The listing builds one solid part. Answer for the finished solid, in the listing's coordinates (mm). Face numbers are marked on the shaded views. A direction names the side the tool comes from. Round coordinates to 2 decimals unless told otherwise and drop trailing zeros.
(1) The mould has two halves that part along Y. Classify the marked faces 1, 2 and 3: +Y half, -Y half, draft (parallel to the pull), parting line (faces both ways), or undercut.
(2) Each of these flat-tipped pins is pushed along its axis until it touches: pin 1 Ø3 at (x, z) = (52, 11) entering from +Y; pin 2 Ø6 at (y, z) = (187, 3) entering from +X; pin 3 Ø6 at (y, z) = (240.5, 4) entering from -X. Where does it stop, or does it pass through?
(3) Find the intervals of material crossed by probe 1 along Y at (x, z) = (65, 4.5); probe 2 along X at (y, z) = (166, 11); probe 3 along X at (y, z) = (217.5, 1.5), in increasing order.
(4) A cutting plane is placed at A-A, the plane y = 163. Give the number of separate pieces and of enclosed holes in the cut face, and give its area (3 significant figures).
(5) For the marked faces 4 and 5, determine the directions among +Z, -Z, +X, -X, +Y, -Y from which every point of the face is accessible in a straight line to the end or side of a thin tool.
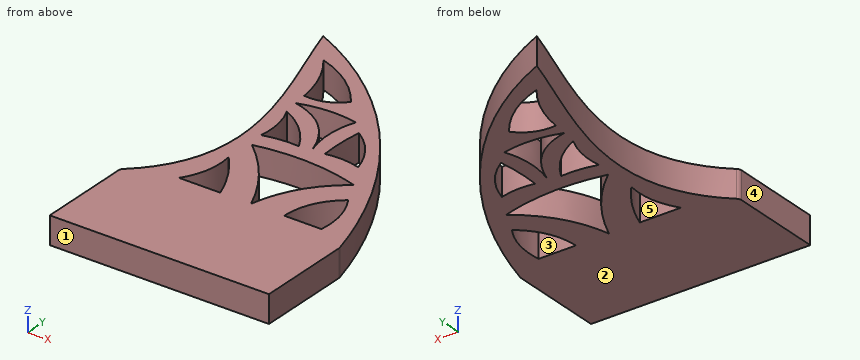
from build123d import *

# Parameters (mm, degrees)
SKETCH1_W           = 101.6
SKETCH1_H           = 152.4
BOSS_EXTRUDE1_DEPTH = 12.7
BOSS_EXTRUDE3_DEPTH = 12.7
FILLET1_R           = 2.54
FILLET2_R           = 5.08
CUT_EXTRUDE1_DEPTH  = 298.570512784


with BuildPart() as part:
    # Sketch1 → Boss-Extrude1 (new body)
    with BuildSketch(Plane.XY):
        with Locations((50.8, 76.2)):
            Rectangle(SKETCH1_W, SKETCH1_H)
    extrude(amount=BOSS_EXTRUDE1_DEPTH)

    # Sketch2 → Boss-Extrude3 (add)
    with BuildSketch(Plane.XY):
        with BuildLine():
            add(Edge.make_bspline(
                [(0, 152.4), (39.790111277, 186.839065643), (12.30975625, 238.845497073), (0, 279.4)],
                knots=[0, 0, 0, 0, 1, 1, 1, 1], degree=3))
            add(Edge.make_bspline(
                [(0, 279.4), (51.286050257, 256.550041835), (87.836892382, 205.957944637), (101.6, 152.4)],
                knots=[0, 0, 0, 0, 1, 1, 1, 1], degree=3))
            Line((101.6, 152.4), (0, 152.4))
        make_face()
        with BuildLine():
            add(Edge.make_bspline(
                [(49.225838487, 233.315766274), (35.641228944, 236.267866949), (22.375615267, 231.937259722)],
                knots=[0, 0, 0, 1, 1, 1], degree=2))
            add(Edge.make_bspline(
                [(48.400350721, 207.535437601), (42.054170901, 227.566198031), (22.375615267, 231.937259722)],
                knots=[0, 0, 0, 1, 1, 1], degree=2))
            add(Edge.make_bspline(
                [(48.400350721, 207.535437601), (44.393568943, 220.734513873), (49.225838487, 233.315766274)],
                knots=[0, 0, 0, 1, 1, 1], degree=2))
        make_face(mode=Mode.SUBTRACT)
        with BuildLine():
            add(Edge.make_bspline(
                [(43.05348098, 206.08803494), (36.239789994, 218.91266054), (23.516066372, 224.861937296)],
                knots=[0, 0, 0, 1, 1, 1], degree=2))
            add(Edge.make_bspline(
                [(23.516066372, 224.861937296), (28.235295407, 215.21927262), (26.605728117, 204.582177714)],
                knots=[0, 0, 0, 1, 1, 1], degree=2))
            add(Edge.make_bspline(
                [(26.605728117, 204.582177714), (34.700432609, 206.792891754), (43.05348098, 206.08803494)],
                knots=[0, 0, 0, 1, 1, 1], degree=2))
        make_face(mode=Mode.SUBTRACT)
        with BuildLine():
            add(Edge.make_bspline(
                [(82.396089655, 183.81371778), (70.6713649, 174.663598784), (70.32777317, 160.02)],
                knots=[0, 0, 0, 1, 1, 1], degree=2))
            Line((70.32777317, 160.02), (87.546521436, 160.02))
            add(Edge.make_bspline(
                [(82.396089655, 183.81371778), (89.339550367, 172.773814043), (87.546521436, 160.02)],
                knots=[0, 0, 0, 1, 1, 1], degree=2))
        make_face(mode=Mode.SUBTRACT)
        with BuildLine():
            add(Edge.make_bspline(
                [(26.980466376, 183.81374211), (28.958775605, 170.837543608), (21.602944743, 160.02)],
                knots=[0, 0, 0, 1, 1, 1], degree=2))
            Line((21.602944743, 160.02), (40.676641776, 160.02))
            add(Edge.make_bspline(
                [(26.980466376, 183.81374211), (36.13847285, 173.175056715), (40.676641776, 160.02)],
                knots=[0, 0, 0, 1, 1, 1], degree=2))
        make_face(mode=Mode.SUBTRACT)
        with BuildLine():
            add(Edge.make_bspline(
                [(54.97708308, 160.02), (46.08347584, 181.54755316), (28.342136903, 196.529802482)],
                knots=[0, 0, 0, 1, 1, 1], degree=2))
            add(Edge.make_bspline(
                [(28.342136903, 196.529802482), (53.017815002, 201.732288521), (77.187204495, 194.363538628)],
                knots=[0, 0, 0, 1, 1, 1], degree=2))
            add(Edge.make_bspline(
                [(54.97708308, 160.02), (59.374728895, 181.400643158), (77.187204495, 194.363538628)],
                knots=[0, 0, 0, 1, 1, 1], degree=2))
        make_face(mode=Mode.SUBTRACT)
        with BuildLine():
            add(Edge.make_bspline(
                [(70.328259561, 206.277457578), (62.361576962, 208.669014941), (54.287141362, 207.109917469)],
                knots=[0, 0, 0, 1, 1, 1], degree=2))
            add(Edge.make_bspline(
                [(54.287141362, 207.109917469), (53.482096811, 217.391663167), (54.97708308, 227.557269012)],
                knots=[0, 0, 0, 1, 1, 1], degree=2))
            add(Edge.make_bspline(
                [(54.97708308, 227.557269012), (66.645859754, 219.852180834), (70.328259561, 206.277457578)],
                knots=[0, 0, 0, 1, 1, 1], degree=2))
        make_face(mode=Mode.SUBTRACT)
        with BuildLine():
            add(Edge.make_bspline(
                [(21.602944743, 238.323137826), (19.95197567, 252.974545225), (11.094737768, 264.601494061)],
                knots=[0, 0, 0, 1, 1, 1], degree=2))
            add(Edge.make_bspline(
                [(11.094737768, 264.601494061), (28.053835186, 259.295838115), (38.412267282, 244.949944056)],
                knots=[0, 0, 0, 1, 1, 1], degree=2))
            add(Edge.make_bspline(
                [(21.602944743, 238.323137826), (31.864782779, 237.284469605), (38.412267282, 244.949944056)],
                knots=[0, 0, 0, 1, 1, 1], degree=2))
        make_face(mode=Mode.SUBTRACT)
    extrude(amount=BOSS_EXTRUDE3_DEPTH)

    # Fillet1
    fillet1_edges = [part.edges().sort_by_distance(p)[0] for p in [
        (101.6, 152.4, 6.35),
        (0, 152.4, 6.35),
    ]]
    fillet(fillet1_edges, radius=FILLET1_R)

    # Fillet2
    fillet2_edges = [part.edges().sort_by_distance(p)[0] for p in [
        (0, 0, 6.35),
        (101.6, 0, 6.35),
    ]]
    fillet(fillet2_edges, radius=FILLET2_R)

    # Sketch4 → Cut-Extrude1 (cut, through all)
    with BuildSketch(Plane.XY.offset(12.7)):
        Polygon((101.519048921, 108.263964199), (0, 108.263964199), (0, 0), (101.6, 0), (101.6, 108.263964199), align=None)
    extrude(amount=-CUT_EXTRUDE1_DEPTH, mode=Mode.SUBTRACT)


solid = part.part
Solutions:
1. face 1: -Y half
1. face 2: draft
1. face 3: undercut
2. pin 1: stops at y = 243.87
2. pin 2: stops at x = 90.66
2. pin 3: stops at x = 12.03
3. probe 1: y = 108.26 to 182.54, 197.27 to 207.43, 217.89 to 227.25
3. probe 2: x = 11.88 to 24.89, 38.32 to 52.27, 56.52 to 70.99, 87.9 to 97.59
3. probe 3: x = 18.88 to 26.16, 34.44 to 43.82, 46.63 to 54.06, 65.27 to 72.1
4. separate pieces: 4
4. enclosed holes: 0
4. area: 677 mm2
5. face 4: +Z, -Z, -X, +Y, -Y
5. face 5: +Z, -Z
